The listing builds one solid part. Answer for the finished solid, in the listing's coordinates (mm). A direction names the side the tool comes from. Give positions to 0.01 mm unless a question says otherwise; leave off trailing zeros. Write each loop counter-clockwise with the first axis right and the second up, starting at its lowest first coordinate (ties: lowest second). Pieces come first, ordered by that corner, then holes. Notation, with made-up numbers: (2, 1) - (39, 1) arc R7 ccw to (39, 5) - close; hole circle Ø10 at (78.5, -6.75). An arc over 180 degrees is marked (long way). Answer as CSV lines item,"result". Start each with the question number.
(1) Straight lines are drawn through the part: probe 1 along X at (y, z) = (-2.5, 1.25); probe 2 along X at (y, z) = (-8.25, 1.25); probe 3 along X at (y, z) = (-4.75, -1.75). For each, find the intervals that lie inside material, in ascending order.
(2) Find section C-C (x = 0). Write down the section's boundary in (y, z) (1 decimal), then the cut area to 3 significant figures.
(3) Each of these flat-tipped pins is pushed along its axis until it touches: pin 1 Ø3 at (y, z) = (-3, 0.5) entering from -X; pin 2 Ø3 at (x, z) = (-40.96, 0) entering from +Y; pin 3 Ø3.5 at (x, z) = (40.96, 0) entering from +Y; pin 4 Ø3 at (y, z) = (-2, -1.5) entering from +X. Where does it stop, or does it pass through?
(4) For faces 5 (the face through (43.42, -13.33, -0.04)), 6 (the face through (-43.688, -3, 0)), 7 (the face through (43.688, -3, 0)), 8 (the face through (43, 0, 0)), 9 (the face through (-41, -11.43, 0)), determine the directions among +Z, -Z, +X, -X, +Y, -Y from which every point of the face is accessible in a straight line to the end or side of a thin tool.
(5) Find section A-A (y = -5.75). Write down the section's boundary in (x, z) (1 decimal), then the cut area to 3 significant figures.
(6) For a pull along X with two mould halves and no side action, classify faces 1 (the face through (-42.099, -5.635, -1.047)), 2 (the face through (43.846, -7.467, 0.044)), 3 (the face through (-43, 0, 0)), 4 (the face through (26.7, -11.3, 0)) as pulls with the +X half, pulls with the -X half, needs draft (parallel to the pull), parting line crosses it, or undercut.
Autodesk Inventor part; units mm, degrees
ref_plane "YZ Plane" through (0, 0, 0) normal (1, 0, 0) x (0, 1, 0)
ref_plane "XZ Plane" through (0, 0, 0) normal (0, 1, 0) x (-1, 0, 0)
ref_plane "XY Plane" through (0, 0, 0) normal (0, 0, 1) x (1, 0, 0)
sketch "Sketch1" plane through (0, 0, 0) normal (0, 0, 1) x (1, 0, 0)
  line L0 (-44.323, 14.2875) -> (44.323, 14.2875)
  line L1 (44.323, 14.2875) -> (44.323, -14.2875)
  line L2 (44.323, -14.2875) -> (-44.323, -14.2875)
  line L3 (-44.323, -14.2875) -> (-44.323, 14.2875)
  point P0 (0, 0)
  dimension "d0" = 88.646
  dimension "d1" = 44.323
  dimension "d2" = 14.2875
  dimension "d3" = 28.575
extrude "Extrusion1" add sketch "Sketch1" along normal mid plane 6.35
sketch "Sketch2" plane through (0, 0, 3.175) normal (0, 0, 1) x (1, 0, 0)
  circle A0 centre (-26.924, 0) radius 11.303
  circle A1 centre (0, 0) radius 11.303
  line L0 (44.323, -14.2875) -> (44.323, 14.2875)
  circle A2 centre (26.924, 0) radius 11.303
  line L1 (-44.323, 14.2875) -> (-44.323, -14.2875)
  line L2 (-44.323, 0) -> (44.323, 0) construction
  line L3 (44.323, 14.2875) -> (-44.323, 14.2875)
  point P0 (0, 0)
  dimension "d6" = 22.606
  dimension "d9" = 22.606
  dimension "d11" = 22.606
  dimension "d14" = 26.924
  dimension "d21" = 88.646
  dimension "d22" = 26.924
  dimension "d50" = 0
sketch "Sketch4" plane through (-44.323, -14.2875, -3.175) normal (-1, 0, 0) x (0, 0, 1)
  line L0 (0, 0) -> (0, 28.575)
  line L1 (6.35, 28.575) -> (6.35, 0)
  line L2 (0, 22.6695) -> (6.35, 22.6695)
  line L3 (6.35, 22.6695) -> (6.35, 5.9055)
  line L4 (6.35, 5.9055) -> (0, 5.9055)
  line L5 (0, 5.9055) -> (0, 22.6695)
  point P0 (3.175, 14.2875)
  dimension "d30" = 8.382
  dimension "d31" = 16.764
extrude "Extrusion3" cut sketch "Sketch4" against normal blind 0.635
mirror "Mirror1" about plane through (0, 0, 0) normal (1, 0, 0) of "Extrusion3"
sketch "Sketch7" plane through (-44.323, -14.2875, 3.175) normal (0, -1, 0) x (1, 0, 0)
  line L0 (30.353, -14.605) -> (58.293, -14.605)
  line L1 (58.293, -14.605) -> (58.293, 8.255)
  line L2 (58.293, 8.255) -> (30.353, 8.255)
  line L3 (30.353, 8.255) -> (30.353, -14.605)
  point P0 (44.323, -3.175)
  dimension "d39" = 27.94
  dimension "d40" = 22.86
  dimension "d41" = 11.43
  dimension "d42" = 13.97
extrude "Extrusion5" [suppressed]
sketch "Sketch8" plane through (0, 0, -3.175) normal (0, 0, -1) x (-1, 0, 0)
  line L0 (-44.323, 14.2875) -> (44.323, 14.2875)
  line L1 (15.6718, 14.2875) -> (-15.6718, 14.2875)
  line L2 (-15.6718, 14.2875) -> (-15.6718, 52.3875)
  line L3 (-15.6718, 52.3875) -> (15.6718, 52.3875)
  line L4 (15.6718, 52.3875) -> (15.6718, 14.2875)
  point P0 (0, 0)
  dimension "d45" = 31.3436
  dimension "d46" = 38.1
  dimension "d47" = 15.6718
extrude "Extrusion6" add sketch "Sketch8" against normal up to surface (6.35 mm away)
extrude "Extrusion7" cut sketch "Sketch2" against normal blind 25.4
sketch "Sketch9" plane through (-15.6718, 52.3875, -3.175) normal (0, 1, 0) x (1, 0, 0)
  line L0 (-28.6512, -6.35) -> (59.9948, -6.35)
  line L1 (3.1718, -6.35) -> (28.1718, -6.35)
  line L2 (28.1718, -6.35) -> (28.1718, -3.175)
  line L3 (28.1718, -3.175) -> (3.1718, -3.175)
  line L4 (3.1718, -3.175) -> (3.1718, -6.35)
  point P0 (15.6718, -3.175)
  dimension "d64" = 3.175
  dimension "d65" = 25
  dimension "d66" = 12.5
extrude "Extrusion8" cut sketch "Sketch9" against normal blind 0.9
sketch "Sketch13" plane through (0, 0, 3.175) normal (0, 0, 1) x (1, 0, 0)
  line L0 (-15.6718, 52.3875) -> (-12.5, 52.3875)
  line L1 (-12.5, 52.3875) -> (12.5, 52.3875)
  line L2 (12.5, 52.3875) -> (15.6718, 52.3875)
  line L3 (15.6718, 52.3875) -> (15.6718, 14.2875)
  line L4 (-15.6718, 14.2875) -> (-15.6718, 52.3875)
  line L5 (-15.6718, 14.2875) -> (-44.323, 14.2875)
  line L6 (44.323, 14.2875) -> (15.6718, 14.2875)
  line L7 (44.323, 8.382) -> (44.323, 14.2875)
  line L8 (-44.323, 14.2875) -> (-44.323, 8.382)
  line L9 (-44.323, 8.382) -> (-43.688, 8.382)
  line L10 (43.688, 8.382) -> (44.323, 8.382)
  line L11 (-43.688, 8.382) -> (-43.688, 0)
  line L12 (-43.688, 8.382) -> (-43.688, -8.382)
  line L13 (-43.688, 0) -> (43.688, 0)
  line L14 (43.688, 8.382) -> (43.688, -8.382)
  line L15 (43.688, 0) -> (43.688, 8.382)
  point P0 (0, 0)
extrude "Extrusion11" cut sketch "Sketch13" against normal through all
sketch "Sketch14" plane through (-43.688, 0, 3.175) normal (0, 1, 0) x (1, 0, 0)
  line L0 (5.461, 6.35) -> (5.461, 0)
  line L1 (0, 6.35) -> (5.461, 6.35)
  line L2 (0, 0) -> (0, 6.35)
  line L3 (5.461, 0) -> (0, 0)
  circle A0 centre (2.7305, 3.175) radius 1.5494
  point P0 (43.688, 3.175)
  dimension "d84" = 3.0988
  dimension "d85" = 5.461
  dimension "d87" = 3.175
  dimension "d88" = 2.7305
  dimension "d98" = 6.35
extrude "Extrusion12" cut sketch "Sketch14" against normal blind 11.43 contours A0
mirror "Mirror3" about plane through (0, 0, 0) normal (1, 0, 0) of "Extrusion12"
thread "Thread3"
thread "Thread4"
fillet "Fillet1" radius 3.175 2 edges at (44.323, -14.2875, 0) (-44.323, -14.2875, 0)
fillet "Fillet3" radius 3.175 2 edges at (-43.688, -8.382, 0) (43.688, -8.382, 0)
equation "\"d9\" = d7"
equation "\"d11\" = d9"
equation "\"d22\" = d14"
equation "\"d87\" = 0.5 * d98"
equation "\"d88\" = 0.5 * d85"
equation "\"d7\" = d6"
properties part number "Tube Holder Halve 3" material "Aluminum 6061-AHC"
Result set:
1,probe 1,"-43.69 to -41.87, -40.04 to -37.95, -15.9 to -11.02, 11.02 to 15.9, 37.95 to 40.04, 41.87 to 43.69"
1,probe 2,"-44.23 to -41.87, -40.04 to -34.65, -19.2 to -7.73, 7.73 to 19.2, 34.65 to 40.04, 41.87 to 44.23"
1,probe 3,"-43.69 to -37.18, -16.67 to -10.26, 10.26 to 16.67, 37.18 to 43.69"
2,outline,"(-14.3, -3.2) - (-11.3, -3.2) - (-11.3, 3.2) - (-14.3, 3.2) - close"
2,area,"19.0 mm^2"
3,pin 1,"x = -43.69"
3,pin 2,"y = -11.43"
3,pin 3,"y = 0"
3,pin 4,"x = 43.69"
4,face 5,"+Z, -Z, +X, -Y"
4,face 6,"+Z, -Z, -X, +Y"
4,face 7,"+Z, -Z, +X, +Y"
4,face 8,"+Z, -Z, +X, -X, +Y"
4,face 9,"+Y"
5,outline,"(-43.7, -3.2) - (-36.7, -3.2) - (-36.7, 3.2) - (-43.7, 3.2) - close; (-17.2, -3.2) - (-9.7, -3.2) - (-9.7, 3.2) - (-17.2, 3.2) - close; (9.7, -3.2) - (17.2, -3.2) - (17.2, 3.2) - (9.7, 3.2) - close; (36.7, -3.2) - (43.7, -3.2) - (43.7, 3.2) - (36.7, 3.2) - close; hole circle Ø3.1 at (-41, 0); hole circle Ø3.1 at (41, 0)"
5,area,"169 mm^2"
6,face 1,"undercut"
6,face 2,"pulls with the +X half"
6,face 3,"needs draft"
6,face 4,"undercut"
